```python
from build123d import *

# Parameters (mm, degrees)
F0_W     = 62.5
F0_H     = 20
F0_R     = 7.5
F0_R_2   = 5
F1_DEPTH = 5.5
F2_DEPTH = 2.5
F3_R     = 2.5
F4_DEPTH = 10


# Not quite as in the source:
# - a feature names something its author has since deleted; it is built from what else it names


with BuildPart() as f1:
    # F0 (on Front) → F1 (new body)
    with BuildSketch(Plane.XZ):
        with Locations((-2, 0)):
            Rectangle(F0_W, F0_H)
        with Locations((-19.25, 0)):
            Circle(F0_R, mode=Mode.SUBTRACT)
        with Locations((17.25, 0)):
            Circle(F0_R_2, mode=Mode.SUBTRACT)
    extrude(amount=F1_DEPTH)

    # F2 (add): a face of the model
    f2_faces = [f1.faces().sort_by_distance(p)[0] for p in [
        (-0.4554491501, -5.5, 0),
    ]]
    extrude(f2_faces, amount=F2_DEPTH)

    # F3 (on face) → F4 (cut)
    with BuildSketch(Plane(origin=(-33.25, 0, 0), x_dir=(0, -1, 0), z_dir=(-1, 0, 0))):
        with Locations((4, 0)):
            Circle(F3_R)
    extrude(amount=-F4_DEPTH, mode=Mode.SUBTRACT)


solid = f1.part
```
Can you work these out from the model? Positions are in its coordinate system, mm. Coordinates: 2 decimals unless noted, no trailing zeros. Write each loop counter-clockwise with the first axis right and the second up, starting at its lowest first coordinate (ties: lowest second). Pieces come first, ordered by that corner, then holes. Notation, with made-up numbers: M 59.25,71.5 L 82.25,71.5 A6 cw 82.25,77.5 Z; hole C 53.5,52.5 d8. An arc over 180 degrees is marked long. Answer as CSV lines item,"result".
Item 1: Imagine slicing it at D-D on x = 17.25. List the corners of the cut face in (y, z) for me.
Geometry results:
outline,"M -8,-10 L 0,-10 L 0,-5 L -8,-5 Z; M -8,5 L 0,5 L 0,10 L -8,10 Z"
Item 2: Imagine slicing it at A-A on y = -4. List the corners of the cut face in (x, z) for me, plus the area to 3 significant figures.
Geometry results:
outline,"M -33.25,-10 L 29.25,-10 L 29.25,10 L -33.25,10 L -33.25,2.5 L -26.32,2.5 A7.5 cw long -26.32,-2.5 L -33.25,-2.5 Z; hole C 17.25,0 d10"
area,"962 mm2"
Item 3: Imagine slicing it at C-C on z = 0. List the corners of the cut face in (x, y) for me.
Geometry results:
outline,"M -33.25,-8 L -26.75,-8 L -26.75,-6.5 L -33.25,-6.5 Z; M -33.25,-1.5 L -26.75,-1.5 L -26.75,0 L -33.25,0 Z; M -11.75,-8 L 12.25,-8 L 12.25,0 L -11.75,0 Z; M 22.25,-8 L 29.25,-8 L 29.25,0 L 22.25,0 Z"
Item 4: Imagine slicing it at B-B on x = -19.25. List the corners of the cut face in (y, z) for me, plus the area to 3 significant figures.
Geometry results:
outline,"M -8,-10 L 0,-10 L 0,-7.5 L -8,-7.5 Z; M -8,7.5 L 0,7.5 L 0,10 L -8,10 Z"
area,"40.0 mm2"
Item 5: We'd pull the mould along Z, two halves only. Please class faces 1 (the flat face through (-33.25, -7, 0)), 2 (the flat face through (-2, -4, 10)), 3 (the cylindrical face through (-29.834, -6.385, 0.751)): +Z half, -Z half, draft (parallel to the pull), parting line (faces both ways), or undercut.
Geometry results:
face 1,"draft"
face 2,"+Z half"
face 3,"undercut"
Item 6: Please list where these lines run through material, in increasing order: line 1 along Z through (x, y) = (-30, -4); line 2 along X through (y, z) = (-2.75, 4); line 3 along X through (y, z) = (-4.25, -3).
Geometry results:
line 1,"z = -10 to -2.5, 2.5 to 10"
line 2,"x = -33.25 to -25.59, -12.91 to 14.25, 20.25 to 29.25"
line 3,"x = -33.25 to -26.12, -12.38 to 13.25, 21.25 to 29.25"
